from build123d import *


with BuildPart() as part:
    # Sketch → Revolution (revolve)
    with BuildSketch(Plane.XZ):
        Polygon((0, 19.92132), (3, 19.92132), (5.12132, 17.8), (5.12132, 14.8), (10.1, 14.8), (11.5, 13.4), (11.5, 7.4), (10.1, 6), (5, 6), (5, 0), (0, 0), align=None)
    revolve(axis=Axis((0, 0, 0), (0, 0, 1)))


solid = part.part
Model file for the job. Use its own axes, mm. A direction names the side the tool comes from. Give positions to 0.01 mm unless a question says otherwise; leave off trailing zeros. Loops run counter-clockwise (first coordinate to the right, second up) from the corner with the lowest first, then second, coordinate; pieces in that order, holes last. Notation, with made-up numbers: (53.25, -12) -> (84.25, -12) arc R27 ccw to (84.25, 13) -> close; hole circle Ø11 at (78, 32). An arc over 180 degrees is marked (long way). Use a Markdown table: item, result. Add a question column.
(1) Slice it at D-D on z = 2. List the corners of the cut face in (x, y).
(2) Tool access for faces 1 (the flat face through (2, 5, 14.8)), 2 (the flat face through (0, 0, 19.921)), 3 (the cylindrical face through (-1.08, -4.88, 2.96)): list every direction of +Z, -Z, +X, -X, +Y, -Y with a clear straight run to the whole face (end or side of a thin tool).
(3) Slice it at C-C on z = 7. List the corners of the cut face in (x, y).
(4) Wall check: line 1 along Y through (x, z) = (2.5, 14.5); line 2 along X through (y, z) = (-0.25, 10.5); line 3 along Z through (x, y) = (-0.5, -8). Give the ranges that are in metal, low to high.
(5) Drop flat-ended pins along their axis: pin 1 Ø3 at (x, z) = (-7.5, 10.5) entering from -Y; pin 2 Ø2 at (y, z) = (7.5, 14) entering from +X; pin 3 Ø1 at (y, z) = (-2, 14.5) entering from -X. Give the stop position or say it passes through.
(6) Slice it at A-A on y = 0. List the corners of the cut face in (x, z).
Filled sheet:
| question | item | result |
|---|---|---|
| 1 | outline | circle Ø10 at (0, 0) |
| 2 | face 1 | +Z |
| 2 | face 2 | +Z, +X, -X, +Y, -Y |
| 2 | face 3 | -Z |
| 3 | outline | circle Ø22.2 at (0, 0) |
| 4 | line 1 | -10.1 to 10.1 |
| 4 | line 2 | -11.5 to 11.5 |
| 4 | line 3 | 6 to 14.8 |
| 5 | pin 1 | y = -9.81 |
| 5 | pin 2 | x = 9.35 |
| 5 | pin 3 | x = -10.72 |
| 6 | outline | (-11.5, 7.4) -> (-10.1, 6) -> (-5, 6) -> (-5, 0) -> (5, 0) -> (5, 6) -> (10.1, 6) -> (11.5, 7.4) -> (11.5, 13.4) -> (10.1, 14.8) -> (5.12, 14.8) -> (5.12, 17.8) -> (3, 19.92) -> (-3, 19.92) -> (-5.12, 17.8) -> (-5.12, 14.8) -> (-10.1, 14.8) -> (-11.5, 13.4) -> close |
